Part print with two shaded views. Sizes in mm from the minimum x, y, z corner. A direction names the side the tool comes from. Give positions to 0.01 mm unless a question says otherwise; leave off trailing zeros. Write each loop counter-clockwise with the first axis right and the second up, starting at its lowest first coordinate (ties: lowest second). Pieces come first, ordered by that corner, then holes. Notation, with made-up numbers: (-15, 7) -> (13, 7) arc R19 ccw to (13, 31) -> close; hole circle Ø11 at (61.5, -12.75). An arc over 180 degrees is marked (long way). Write item = value, one per line. Start each with the question number.
Q1. Tool access for the marked faces 1 and 2: list every direction of +Z, -Z, +X, -X, +Y, -Y with a clear straight run to the whole face (end or side of a thin tool).
Q2. Saw through at A-A, the plane y = 7.75. List the corners of the cut face in (x, z), then the cut area to 3 significant figures.
Q3. Saw through at C-C, the plane z = 55. List the corners of the cut face in (x, y).
Q4. Wall check: line 1 (X direction, y = 7, z = 43); line 2 (Z direction, x = 22, y = 2.75); line 3 (Y direction, x = 11.5, z = 57.5). Give the ranges that are in metal, low to high.
Q5. Drop a flat-ended pin along its axis: P1, Ø6, axis at x = 34.5, z = 57.5, coming from the +Y side. Give the stop position or say it passes through.
Q6. Saw through at B-B, the plane x = 32.5. List the corners of the cut face in (y, z).
Q7. Mould opens along Z. For the marked faces 3, 4 and 5 say: pulls with the +Z half, pulls with the -Z half, needs draft (parallel to the pull), parting line crosses it, or undercut.
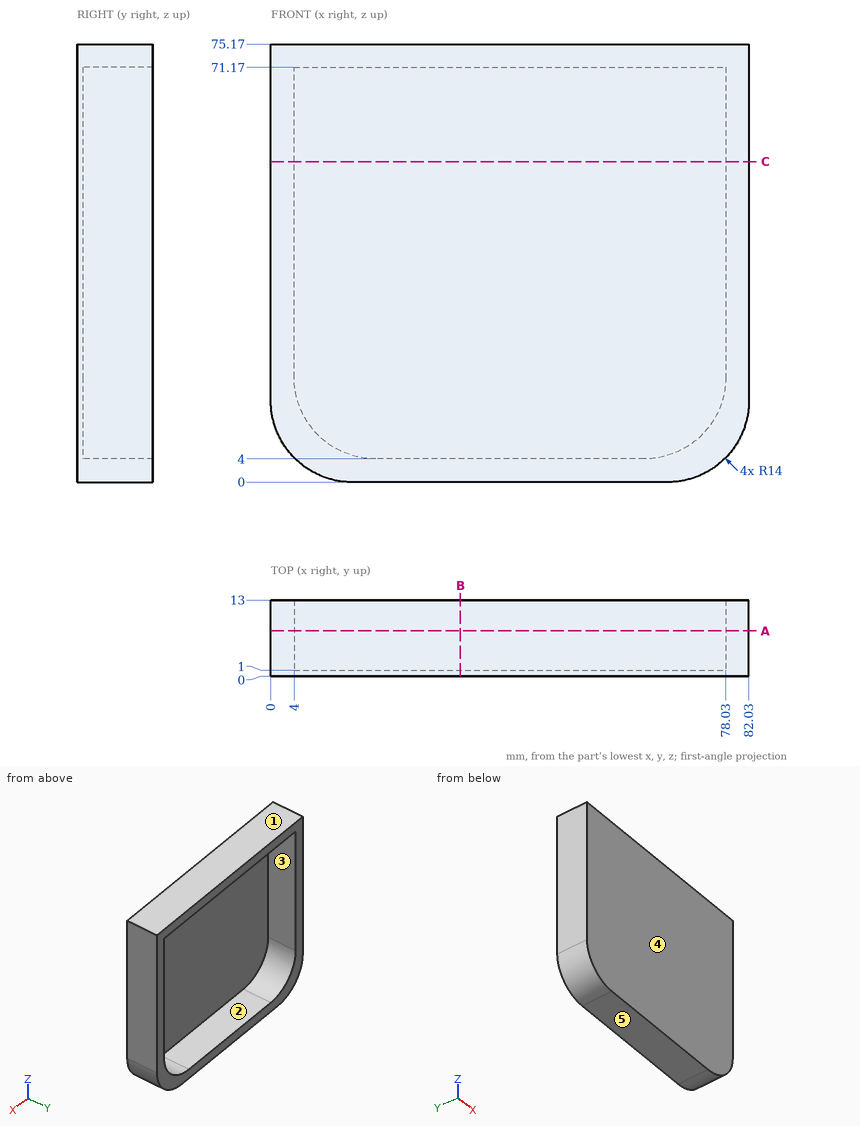
Report:
q1.face_1 = +Z, +X, -X, +Y, -Y
q1.face_2 = +Y
q2.outline = (0, 14) arc R14 ccw to (14, 0) -> (68.03, 0) arc R14 ccw to (82.03, 14) -> (82.03, 75.17) -> (0, 75.17) -> close; hole (4, 18) arc R14 ccw to (18, 4) -> (64.03, 4) arc R14 ccw to (78.03, 18) -> (78.03, 71.17) -> (4, 71.17) -> close
q2.area = 1,190 mm2
q3.outline = (0, 0) -> (82.03, 0) -> (82.03, 13) -> (78.03, 13) -> (78.03, 1) -> (4, 1) -> (4, 13) -> (0, 13) -> close
q4.line_1 = 0 to 4, 78.03 to 82.03
q4.line_2 = 0 to 4, 71.17 to 75.17
q4.line_3 = 0 to 1
q5.P1 = 1
q6.outline = (0, 0) -> (13, 0) -> (13, 4) -> (1, 4) -> (1, 71.17) -> (13, 71.17) -> (13, 75.17) -> (0, 75.17) -> close
q7.face_3 = undercut
q7.face_4 = needs draft
q7.face_5 = pulls with the -Z half
